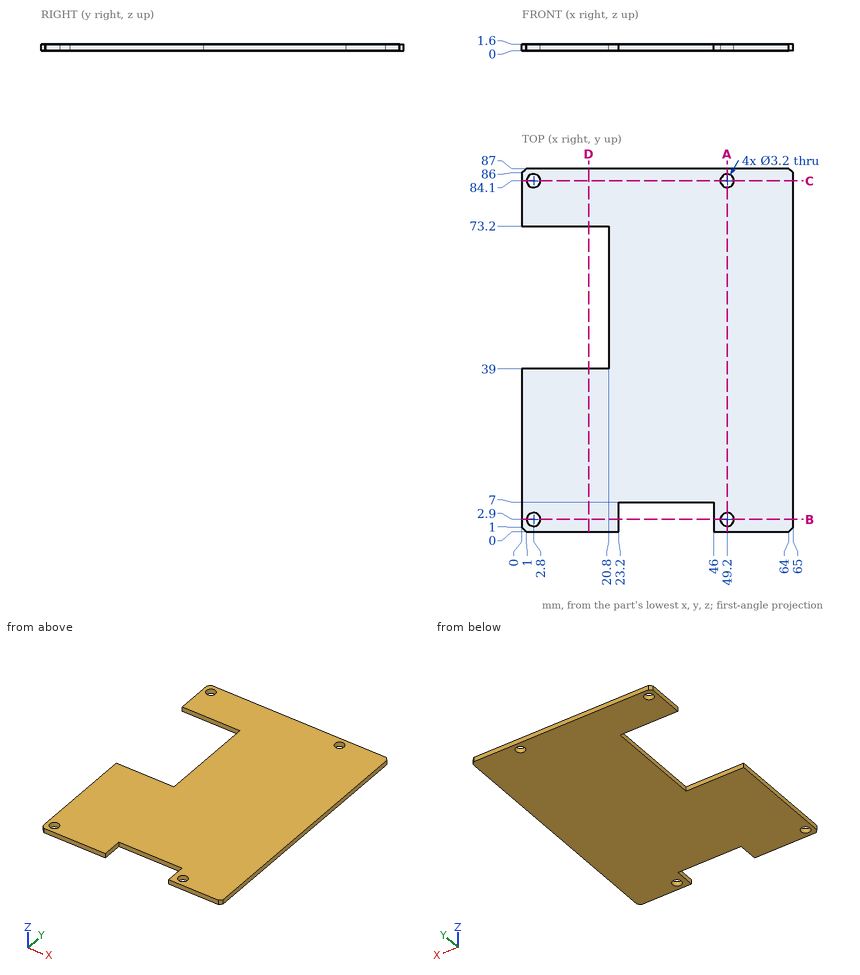
The figure shows three views and two pictorial views of one solid part (mm, origin at its lowest corner). Answer the questions. Round coordinates to 2 decimals unless told otherwise and drop trailing zeros. Loops run counter-clockwise (first coordinate to the right, second up) from the corner with the lowest first, then second, coordinate; pieces in that order, holes last. Notation, with made-up numbers: (88, -37.75) - (113, -37.75) arc R35 cw to (113, -4.75) - close; hole circle Ø4 at (81, 40.5). An arc over 180 degrees is marked (long way). One line per question, with ' | ' between items. Start each with the question number.
Q1. Find the intervals of material crossed by L1, parallel to Y at x = 49.2, z = 0.95; L2, parallel to X at y = 84.1, z = 0.45; L3, parallel to Y at x = 2.8, z = 0.4, in increasing order.
Q2. Section A-A on x = 49.2 is taken. Give the vertices of the cut face in (y, z).
Q3. Section B-B on y = 2.9 is taken. Give the vertices of the cut face in (x, z), plus the area to 3 significant figures.
Q4. Flat-ended cylindrical pins translate along their axes: pin 1 (2.5 mm diameter, centred on x = 2.8, y = 2.9, fed in from -Z); pin 2 (0.8 mm diameter, centred on x = 33.5, z = 1, fed in from -Y); pin 3 (0.8 mm diameter, centred on y = 64, z = 0.5, fed in from -X). Find the tip coordinate at first contact, or state that the pin passes through.
Q5. Section D-D on x = 16 is taken. Give the vertices of the cut face in (y, z).
Q6. Section C-C on y = 84.1 is taken. Give the vertices of the cut face in (x, z).
Established:
1) L1: 0 to 1.3, 4.5 to 82.5, 85.7 to 87 | L2: 0 to 1.2, 4.4 to 47.6, 50.8 to 65 | L3: 0 to 1.3, 4.5 to 39, 73.2 to 82.5, 85.7 to 87
2) outline: (0, 0) - (1.3, 0) - (1.3, 1.6) - (0, 1.6) - close; (4.5, 0) - (82.5, 0) - (82.5, 1.6) - (4.5, 1.6) - close; (85.7, 0) - (87, 0) - (87, 1.6) - (85.7, 1.6) - close
3) outline: (0, 0) - (1.2, 0) - (1.2, 1.6) - (0, 1.6) - close; (4.4, 0) - (23.2, 0) - (23.2, 1.6) - (4.4, 1.6) - close; (46, 0) - (47.6, 0) - (47.6, 1.6) - (46, 1.6) - close; (50.8, 0) - (65, 0) - (65, 1.6) - (50.8, 1.6) - close | area: 57.3 mm²
4) pin 1: through | pin 2: y = 7 | pin 3: x = 20.8
5) outline: (0, 0) - (39, 0) - (39, 1.6) - (0, 1.6) - close; (73.2, 0) - (87, 0) - (87, 1.6) - (73.2, 1.6) - close
6) outline: (0, 0) - (1.2, 0) - (1.2, 1.6) - (0, 1.6) - close; (4.4, 0) - (47.6, 0) - (47.6, 1.6) - (4.4, 1.6) - close; (50.8, 0) - (65, 0) - (65, 1.6) - (50.8, 1.6) - close
